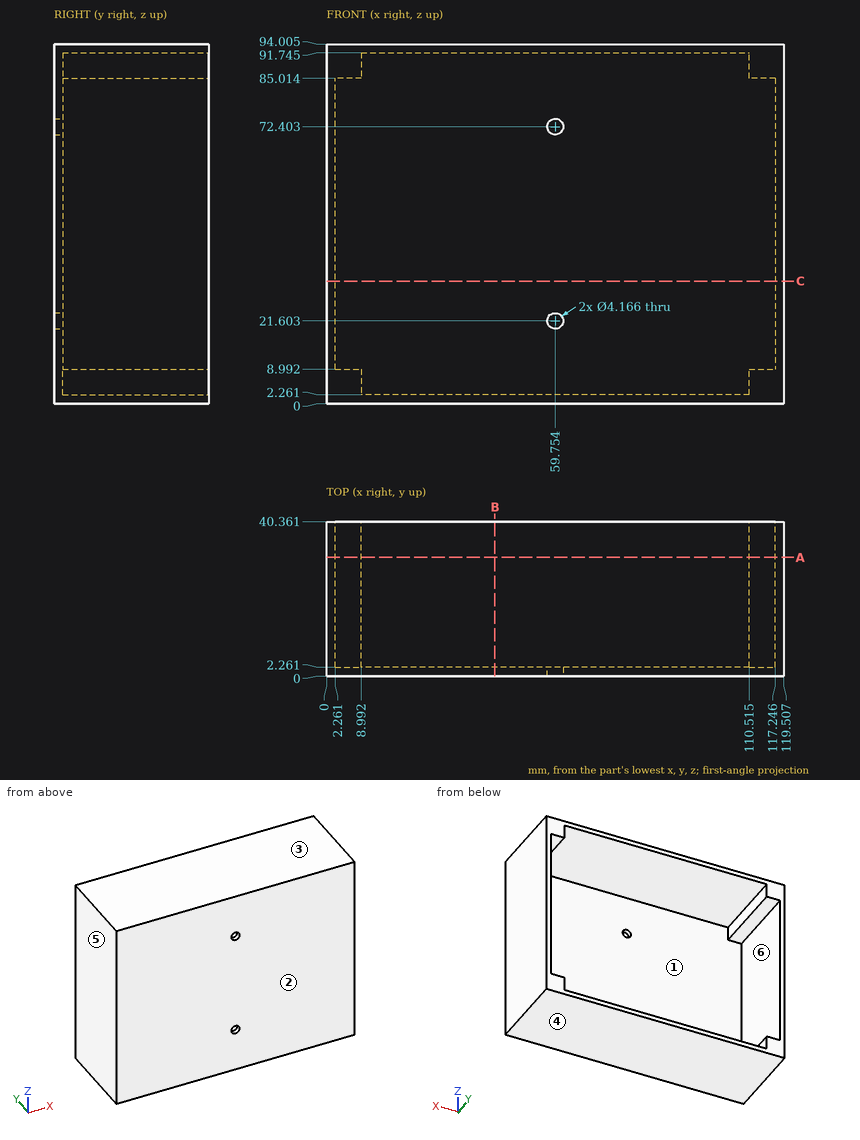
For this review, use the dimensioned drawing (mm, ordinates from the lowest corner) and the shaded views. A direction names the side the tool comes from. Give positions to 0.01 mm unless a question says otherwise; leave off trailing zeros. Write each loop counter-clockwise with the first axis right and the second up, starting at its lowest first coordinate (ties: lowest second). Pieces come first, ordered by that corner, then holes. Notation, with made-up numbers: M -12,24 L 39,24 A24 cw 39,55 Z; hole C 20,17 d1. An arc over 180 degrees is marked long. Write item = value, one per line. Start each with the question number.
Q1. Clearance check with a flat-ended pin moving along its axis: pin 1 (10 mm diameter, centred on x = 88.5, z = 23, fed in from +Y). State where the tip first meets the part, or that it passes through.
Q2. We need section A-A (y = 31). State the section outline as (x, z) points (1 decimal).
Q3. For line 1 (Z direction, x = 66, y = 36) (1 decimal); line 2 (X direction, y = 33, z = 4.5) (1 decimal); line 3 (X direction, y = 3, z = 57.5), list the stretches that pass through material, from the lowest coordinate up.
Q4. We need section B-B (x = 44). State the section outline as (y, z) points (1 decimal).
Q5. Mouldability with a two-part tool opening along Z and no side actions: class the marked faces 1, 2, 3 and 4 as released by +Z, released by -Z, zero draft, split by the parting line, or undercut.
Q6. We need section C-C (z = 32). State the section outline as (x, y) points.
Q7. Machinability: for the marked faces 5 and 6, which of the approach directions +Z, -Z, +X, -X, +Y, -Y give a long, thin tool a straight path to every point of the face, cutting with its end or side? Answer none if there is none.
Result set:
q1.pin_1 = 2.26
q2.outline = M 0,0 L 119.5,0 L 119.5,94 L 0,94 Z; hole M 2.3,9 L 9,9 L 9,2.3 L 110.5,2.3 L 110.5,9 L 117.2,9 L 117.2,85 L 110.5,85 L 110.5,91.7 L 9,91.7 L 9,85 L 2.3,85 Z
q3.line_1 = 0 to 2.3, 91.7 to 94
q3.line_2 = 0 to 9, 110.5 to 119.5
q3.line_3 = 0 to 2.26, 117.25 to 119.51
q4.outline = M 0,0 L 40.4,0 L 40.4,2.3 L 2.3,2.3 L 2.3,91.7 L 40.4,91.7 L 40.4,94 L 0,94 Z
q5.face_1 = undercut
q5.face_2 = zero draft
q5.face_3 = released by +Z
q5.face_4 = released by -Z
q6.outline = M 0,0 L 119.51,0 L 119.51,40.36 L 117.25,40.36 L 117.25,2.26 L 2.26,2.26 L 2.26,40.36 L 0,40.36 Z
q7.face_5 = +Z, -Z, -X, +Y, -Y
q7.face_6 = +Y
